```python
from build123d import *

# Parameters (mm, degrees)
F0_W     = 533.4
F0_H     = 381
F1_DEPTH = 12.7
F5_W     = 25.4
F5_H     = 6.35
F5_W_2   = 6.35
F5_H_2   = 25.4
F5_R     = 3.175
F5_R_2   = 4.28625
F5_R_3   = 4.2926
F5_W_3   = 63.5
F5_H_3   = 88.9
F4_R     = 4.28625
F4_W     = 25.4
F4_H     = 6.35
F4_R_2   = 4.2926
F4_W_2   = 6.35
F4_H_2   = 25.4
F4_W_3   = 63.5
F4_H_3   = 88.9
F6_DEPTH = 12.701


# Not quite as in the source:
# - a feature of the source that left no trace in its solid (it failed there, or was rolled back) is left out


with BuildPart() as f1:
    # F0 (on Top) → F1 (new body)
    with BuildSketch(Plane.XY):
        Rectangle(F0_W, F0_H)
    extrude(amount=F1_DEPTH)

    # F5 (on face) + F4 (on face) → F6 (cut, through all)
    with BuildSketch(Plane.XY.offset(12.7)):
        with Locations((0, -24.4856)):
            Rectangle(F5_W, F5_H)
        with Locations((87.9475, -88.6206)):
            Rectangle(F5_W_2, F5_H_2)
        with Locations((0, -152.7556)):
            Rectangle(F5_W, F5_H)
        with Locations((-87.9475, -88.6206)):
            Rectangle(F5_W_2, F5_H_2)
        with Locations((-103.575, 20.447)):
            Circle(F5_R)
        with Locations((-103.575, -15.113)):
            Circle(F5_R)
        with Locations((220.6625, -67.183)):
            Circle(F5_R)
        with Locations((220.6625, -109.093)):
            Circle(F5_R)
        with Locations((100.4, 20.447)):
            Circle(F5_R)
        with Locations((100.4, -21.463)):
            Circle(F5_R)
        with Locations((118.4275, -57.023)):
            Rectangle(F5_W_2, F5_H_2)
        with Locations((195.8975, -57.023)):
            Rectangle(F5_W_2, F5_H_2)
        with Locations((-128.6256, -135.89)):
            Circle(F5_R_2)
        with Locations((0, -11.938)):
            Rectangle(F5_W, F5_H)
        with Locations((-162.4810314, 41.0845)):
            Circle(F5_R_3)
        with Locations((-162.4810314, 79.0575)):
            Circle(F5_R_3)
        with Locations((-108.0289686, 41.0845)):
            Circle(F5_R_3)
        with Locations((-81.28, 40.767)):
            Rectangle(F5_W_2, F5_H_2)
        with Locations((-108.0289686, 79.0575)):
            Circle(F5_R_3)
        with Locations((-204.8256, 107.95)):
            Rectangle(F5_W_3, F5_H_3)
        with Locations((-156.810075, 106.3625)):
            Circle(F5_R_3)
        with Locations((-128.6256, 141.9225)):
            Circle(F5_R_2)
        with Locations((-58.0445372, 106.3625)):
            Circle(F5_R_2)
        with Locations((81.28, 40.767)):
            Rectangle(F5_W_2, F5_H_2)
        with Locations((108.0289686, 41.0845)):
            Circle(F5_R_3)
        with Locations((0, 94.2975)):
            Rectangle(F5_W, F5_H)
        with Locations((108.0289686, 79.0575)):
            Circle(F5_R_3)
        with Locations((162.4810314, 41.0845)):
            Circle(F5_R_3)
        with Locations((162.4810314, 79.0575)):
            Circle(F5_R_3)
        with Locations((58.0445372, 106.3625)):
            Circle(F5_R_2)
        with Locations((128.6256, 141.9225)):
            Circle(F5_R_2)
        with Locations((156.810075, 106.3625)):
            Circle(F5_R_3)
        with Locations((204.8256, 107.95)):
            Rectangle(F5_W_3, F5_H_3)
    with BuildSketch(Plane.XY.offset(12.7)):
        with Locations((-133.35, 173.99)):
            Circle(F4_R)
        with Locations((0, 173.99)):
            Circle(F4_R)
        with Locations((133.35, 173.99)):
            Circle(F4_R)
        with Locations((250.19, 0)):
            Circle(F4_R)
        with Locations((-250.19, 0)):
            Circle(F4_R)
        with Locations((0, -173.99)):
            Circle(F4_R)
        with Locations((133.35, -173.99)):
            Circle(F4_R)
        with Locations((-133.35, -173.99)):
            Circle(F4_R)
        with Locations((-128.6256, -135.89)):
            Circle(F4_R)
        with Locations((0, -11.938)):
            Rectangle(F4_W, F4_H)
        with Locations((-162.4810314, 41.0845)):
            Circle(F4_R_2)
        with Locations((-162.4810314, 79.0575)):
            Circle(F4_R_2)
        with Locations((-108.0289686, 41.0845)):
            Circle(F4_R_2)
        with Locations((-81.28, 40.767)):
            Rectangle(F4_W_2, F4_H_2)
        with Locations((-108.0289686, 79.0575)):
            Circle(F4_R_2)
        with Locations((-204.8256, 107.95)):
            Rectangle(F4_W_3, F4_H_3)
        with Locations((-156.810075, 106.3625)):
            Circle(F4_R_2)
        with Locations((-128.6256, 141.9225)):
            Circle(F4_R)
        with Locations((-58.0445372, 106.3625)):
            Circle(F4_R)
        with Locations((81.28, 40.767)):
            Rectangle(F4_W_2, F4_H_2)
        with Locations((108.0289686, 41.0845)):
            Circle(F4_R_2)
        with Locations((0, 94.2975)):
            Rectangle(F4_W, F4_H)
        with Locations((108.0289686, 79.0575)):
            Circle(F4_R_2)
        with Locations((162.4810314, 41.0845)):
            Circle(F4_R_2)
        with Locations((162.4810314, 79.0575)):
            Circle(F4_R_2)
        with Locations((58.0445372, 106.3625)):
            Circle(F4_R)
        with Locations((128.6256, 141.9225)):
            Circle(F4_R)
        with Locations((156.810075, 106.3625)):
            Circle(F4_R_2)
        with Locations((204.8256, 107.95)):
            Rectangle(F4_W_3, F4_H_3)
    extrude(amount=-F6_DEPTH, mode=Mode.SUBTRACT)


solid = f1.part
```
Build history of the part. All positions in model axes, mm. Round coordinates to 2 decimals unless told otherwise and drop trailing zeros. Write each loop counter-clockwise with the first axis right and the second up, starting at its lowest first coordinate (ties: lowest second). Pieces come first, ordered by that corner, then holes. Notation, with made-up numbers: (65.25, -31) - (118.25, -31) arc R3 cw to (118.25, -27) - close; hole circle Ø4 at (-9, 70.5). An arc over 180 degrees is marked (long way). Write each question's results on one line, items separated by ' | '. Start each with the question number.
Item 1: Saw through at C-C (z = 10). State how many separate pieces and enclosed holes the cut face has, and give its area (3 significant figures).
Item 2: Wall check: L1, parallel to Y at x = 9.5, z = 9.5; L2, parallel to X at y = 122, z = 4.75; L3, parallel to Y at x = 130.5, z = 1. Give the ranges that are in metal, low to high. Write a range as [from, to].
Item 3: Mould opens along X. For faces 1 (the face through (-4, -190.5, 6)), 2 (the face through (192.722, -57, 6)) say: pulls with the +X half, pulls with the -X half, needs draft (parallel to the pull), parting line crosses it, or undercut.
Item 4: Saw through at A-A (y = -57). Write the cut outline in (x, z).
Item 5: Saw through at B-B (x = 231). Write the cut outline in (y, z), and give its area (3 significant figures).
Item 6: Drop a flat-ended pin along its axis: P1, Ø7.5, axis at x = -162.48, y = 41.08, coming from the -Z side. Give the stop position or say it passes through.
Results are:
1) separate pieces: 1 | enclosed holes: 41 | area: 189,000 mm²
2) L1: y = [-190.5, -155.93], [-149.58, -27.66], [-21.31, -15.11], [-8.76, 91.12], [97.47, 190.5] | L2: x = [-266.7, -236.58], [-173.08, 173.08], [236.58, 266.7] | L3: y = [-190.5, -177.19], [-170.79, 138.07], [145.78, 170.79], [177.19, 190.5]
3) face 1: needs draft | face 2: undercut
4) outline: (-266.7, 0) - (115.25, 0) - (115.25, 12.7) - (-266.7, 12.7) - close; (121.6, 0) - (192.72, 0) - (192.72, 12.7) - (121.6, 12.7) - close; (199.07, 0) - (266.7, 0) - (266.7, 12.7) - (199.07, 12.7) - close
5) outline: (-190.5, 0) - (63.5, 0) - (63.5, 12.7) - (-190.5, 12.7) - close; (152.4, 0) - (190.5, 0) - (190.5, 12.7) - (152.4, 12.7) - close | area: 3,710 mm²
6) P1: passes through
